Geometry check sheet. Reference: the model listing, model coordinates, mm. Face numbers are marked on the shaded views. A direction names the side the tool comes from. Give positions to 0.01 mm unless a question says otherwise; leave off trailing zeros. Loops run counter-clockwise (first coordinate to the right, second up) from the corner with the lowest first, then second, coordinate; pieces in that order, holes last. Notation, with made-up numbers: (-12.75, 21.5) -> (13.25, 21.5) arc R37 ccw to (13.25, 58.5) -> close; hole circle Ø1 at (71, 2.25). An arc over 180 degrees is marked (long way). One line per question, with ' | ' between items.
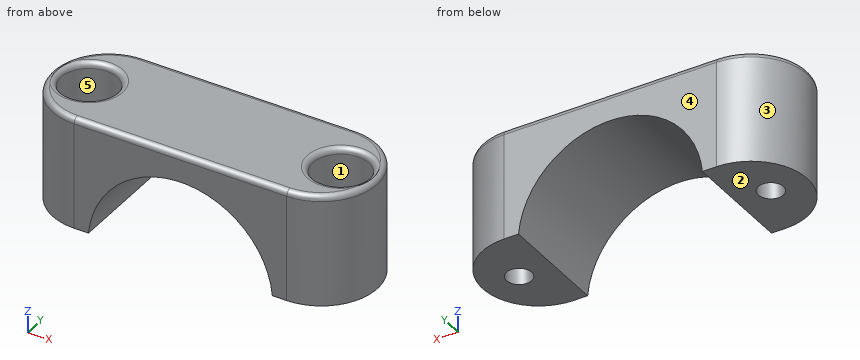
Autodesk Inventor part; units mm, degrees
ref_plane "YZ Plane" through (0, 0, 0) normal (1, 0, 0) x (0, 1, 0)
ref_plane "XZ Plane" through (0, 0, 0) normal (0, 1, 0) x (-1, 0, 0)
ref_plane "XY Plane" through (0, 0, 0) normal (0, 0, 1) x (1, 0, 0)
sketch "Sketch1" plane through (0, 0, 0) normal (0, 0, 1) x (1, 0, 0)
  line L0 (19, 10) -> (-19, 10)
  arc A0 (19, -10) -> (19, 10) centre (19, 0) ccw
  line L1 (-19, -10) -> (19, -10)
  arc A1 (-19, 10) -> (-19, -10) centre (-19, 0) ccw
  circle A2 centre (22.5, 0) radius 2.25
  circle A3 centre (-22.5, 0) radius 2.25
  point P0 (0, 0)
extrude "Extrusion1" add sketch "Sketch1" along normal blind 20 contours A0 L1 A1 L0 | A2 | A3
sketch "Sketch2" plane through (-19, -10, 0) normal (0, -1, 0) x (1, 0, 0)
  arc A0 (3, 0) -> (35, 0) centre (19, 0) ccw
  line L0 (3, 0) -> (0, 0)
  line L1 (0, -40) -> (0, 0)
  line L2 (0, -40) -> (38, -40)
  line L3 (38, -40) -> (38, 0)
  line L4 (38, 0) -> (35, 0)
  circle A1 centre (19, 0) radius 16
  line L5 (0, 0) -> (38, 0)
  line L6 (38, 0) -> (38, 20)
  line L7 (0, 20) -> (38, 20)
  line L8 (0, 0) -> (0, 20)
  point P0 (19, 0)
  point P1 (3, 0)
  point P2 (35, 0)
extrude "Extrusion2" cut sketch "Sketch2" against normal through all contours A1 L5
sketch "Sketch3" plane through (0, 0, 20) normal (0, 0, 1) x (1, 0, 0)
  arc A0 (-19, 10) -> (-19, -10) centre (-19, 0) ccw
  line L0 (-19, -10) -> (19, -10)
  arc A1 (19, -10) -> (19, 10) centre (19, 0) ccw
  line L1 (19, 10) -> (-19, 10)
  line L2 (-16, -10.4231) -> (-16, -76.7035)
  arc A2 (-19, 10) -> (-19, -10) centre (-19, 0) ccw
  line L3 (-29, 0) -> (-16, 0)
  circle A3 centre (-22.5, 0) radius 2.25
  line L4 (19, 10) -> (-19, 10)
  line L5 (0, 10) -> (0, -10)
  circle A4 centre (22.5, 0) radius 2.25
  line L6 (-22.5, 0) -> (-26, 0)
  line L7 (-26, 2.0207) -> (-22.5, 4.0415)
  line L8 (-22.5, 4.0415) -> (-19, 2.0207)
  line L9 (-19, 2.0207) -> (-19, -2.0207)
  line L10 (-19, -2.0207) -> (-22.5, -4.0415)
  line L11 (-22.5, -4.0415) -> (-26, -2.0207)
  line L12 (-26, -2.0207) -> (-26, 2.0207)
  line L13 (26, 2.0207) -> (22.5, 4.0415)
  line L14 (22.5, 4.0415) -> (19, 2.0207)
  line L15 (19, 2.0207) -> (19, -2.0207)
  line L16 (19, -2.0207) -> (22.5, -4.0415)
  line L17 (22.5, -4.0415) -> (26, -2.0207)
  line L18 (26, -2.0207) -> (26, 2.0207)
  point P0 (0, 0)
  dimension "d4" = 4.5
  dimension "d5" = 3.5
extrude "Extrusion3" [suppressed]
extrude "Extrusion4" cut sketch "Sketch3" against normal blind 5.5 contours L3 A3 | L3 A3 | A3 L3 L12 L7 L8 L9 | L3 L9 L10 L11 L12 A3 | A4 | L18 L17 L16 L15 L14 L13
extrude "Extrusion5" cut sketch "Sketch3" against normal through all contours L3 A3 | L3 A3 | A4
sketch "Sketch4" plane through (0, 0, 20) normal (0, 0, 1) x (1, 0, 0)
  line L0 (19, 2.0207) -> (22.5, 4.0415)
  line L1 (22.5, 4.0415) -> (26, 2.0207)
  line L2 (26, 2.0207) -> (26, -2.0207)
  line L3 (26, -2.0207) -> (22.5, -4.0415)
  line L4 (22.5, -4.0415) -> (19, -2.0207)
  line L5 (19, -2.0207) -> (19, 2.0207)
  line L6 (-19, -2.0207) -> (-22.5, -4.0415)
  line L7 (-22.5, -4.0415) -> (-26, -2.0207)
  line L8 (-26, -2.0207) -> (-26, 2.0207)
  line L9 (-26, 2.0207) -> (-22.5, 4.0415)
  line L10 (-22.5, 4.0415) -> (-19, 2.0207)
  line L11 (-19, 2.0207) -> (-19, -2.0207)
  arc A0 (-19, 10) -> (-19, -10) centre (-19, 0) ccw
  line L12 (-19, -10) -> (19, -10)
  arc A1 (19, -10) -> (19, 10) centre (19, 0) ccw
  line L13 (19, 10) -> (-19, 10)
  point P0 (0, 0)
extrude "Extrusion6" add sketch "Sketch4" along normal blind 1.5
sketch "Sketch5" plane through (0, 0, 0) normal (0, 0, -1) x (-1, 0, 0)
  circle A0 centre (-22.5, 0) radius 2.25
  line L0 (-16, -10) -> (-16, 10)
  line L1 (-19, 10) -> (-16, 10)
  arc A1 (-19, 10) -> (-19, -10) centre (-19, 0) ccw
  line L2 (-16, -10) -> (-19, -10)
  circle A2 centre (22.5, 0) radius 2.25
  line L3 (16, 10) -> (16, -10)
  line L4 (19, -10) -> (16, -10)
  arc A3 (19, -10) -> (19, 10) centre (19, 0) ccw
  line L5 (16, 10) -> (19, 10)
  point P0 (0, 0)
extrude "Extrusion7" cut sketch "Sketch5" against normal blind 0.5
sketch "Sketch6" plane through (0, -10, 0) normal (0, -1, 0) x (1, 0, 0)
  line L0 (-19, 0.5) -> (-19, 21.5)
  line L1 (-19, 0.5) -> (-16, 0.5)
  line L2 (-16, 0.5) -> (-16, 0)
  arc A0 (16, 0) -> (-16, 0) centre (0, 0) ccw
  line L3 (16, 0) -> (16, 0.5)
  line L4 (16, 0.5) -> (19, 0.5)
  line L5 (19, 0.5) -> (19, 21.5)
  arc A1 (16, 0) -> (-16, 0) centre (0, 0) ccw
  line L6 (0, 16) -> (0, 16.5)
  circle A2 centre (0, 0) radius 16.5
  line L7 (-19, 21.5) -> (19, 21.5)
  point P0 (0, 0)
  point P1 (16.4924, 0.5)
  point P2 (-16.4924, 0.5)
  dimension "d17" = 0.5
extrude "Extrusion8" cut sketch "Sketch6" against normal through all contours A2 L6 A0 L2 L1 | A2 L4 L3 A0 L6
sketch "Sketch7" plane through (0, 0, 21.5) normal (0, 0, 1) x (1, 0, 0)
  circle A0 centre (-22.5, 0) radius 2.25
  line L0 (-22.5, -4.0415) -> (-26, -2.0207)
  line L1 (-19, -2.0207) -> (-22.5, -4.0415)
  line L2 (-19, 2.0207) -> (-19, -2.0207)
  line L3 (-22.5, 4.0415) -> (-19, 2.0207)
  line L4 (-26, 2.0207) -> (-22.5, 4.0415)
  line L5 (-26, -2.0207) -> (-26, 2.0207)
  circle A1 centre (22.5, 0) radius 2.25
  line L6 (22.5, 4.0415) -> (26, 2.0207)
  line L7 (19, 2.0207) -> (22.5, 4.0415)
  line L8 (19, -2.0207) -> (19, 2.0207)
  line L9 (22.5, -4.0415) -> (19, -2.0207)
  line L10 (26, -2.0207) -> (22.5, -4.0415)
  line L11 (26, 2.0207) -> (26, -2.0207)
  point P0 (0, 0)
extrude "Extrusion9" cut sketch "Sketch7" against normal blind 15
sketch "Sketch8" plane through (0, 0, 21.5) normal (0, 0, 1) x (1, 0, 0)
  line L0 (-19, -10) -> (19, -10)
  arc A0 (19, -10) -> (19, 10) centre (19, 0) ccw
  line L1 (19, 10) -> (-19, 10)
  arc A1 (-19, 10) -> (-19, -10) centre (-19, 0) ccw
  line L2 (-19, -2.0207) -> (-22.5, -4.0415)
  line L3 (-22.5, -4.0415) -> (-26, -2.0207)
  line L4 (-26, -2.0207) -> (-26, 2.0207)
  line L5 (-26, 2.0207) -> (-22.5, 4.0415)
  line L6 (-22.5, 4.0415) -> (-19, 2.0207)
  line L7 (-19, 2.0207) -> (-19, -2.0207)
  line L8 (19, 2.0207) -> (22.5, 4.0415)
  line L9 (22.5, 4.0415) -> (26, 2.0207)
  line L10 (26, 2.0207) -> (26, -2.0207)
  line L11 (26, -2.0207) -> (22.5, -4.0415)
  line L12 (22.5, -4.0415) -> (19, -2.0207)
  line L13 (19, -2.0207) -> (19, 2.0207)
  circle A2 centre (-22.5, 0) radius 2.25
  circle A3 centre (22.5, 0) radius 2.25
  circle A4 centre (-22.5, 0) radius 5
  circle A5 centre (22.5, 0) radius 5
  point P0 (0, 0)
  dimension "d22" = 10
  dimension "d23" = 10
extrude "Extrusion10" cut sketch "Sketch8" against normal blind 11 contours L2 L3 L4 L5 L6 L7 | L8 L9 L10 L11 L12 L13 | A2 | A3 | A4 | A5
fillet "Fillet2" radius 1 6 edges at (0, -10, 21.5) (29, 0, 21.5) (0, 10, 21.5) (-29, 0, 21.5) (-27.5, 0, 21.5) (17.5, 0, 21.5)
sketch "Szkic9" plane through (0, 0, 6.5) normal (0, 0, 1) x (1, 0, 0)
  line L0 (-19, 2.0207) -> (-19, -2.0207)
  line L1 (-22.5, 4.0415) -> (-19, 2.0207)
  line L2 (-26, 2.0207) -> (-22.5, 4.0415)
  line L3 (-26, -2.0207) -> (-26, 2.0207)
  line L4 (-22.5, -4.0415) -> (-26, -2.0207)
  line L5 (-19, -2.0207) -> (-22.5, -4.0415)
  circle A0 centre (-22.5, 0) radius 2.25
  line L6 (19, -2.0207) -> (19, 2.0207)
  line L7 (22.5, -4.0415) -> (19, -2.0207)
  line L8 (26, -2.0207) -> (22.5, -4.0415)
  line L9 (26, 2.0207) -> (26, -2.0207)
  line L10 (22.5, 4.0415) -> (26, 2.0207)
  line L11 (19, 2.0207) -> (22.5, 4.0415)
  circle A1 centre (22.5, 0) radius 2.25
  point P0 (0, 0)
extrude "Wyciągnięcie proste11" cut sketch "Szkic9" against normal blind 1
sketch "Szkic10" plane through (0, 0, 0.5) normal (0, 0, -1) x (-1, 0, 0)
  line L0 (-16.4924, -10) -> (-16.4924, 10)
  line L1 (-19, 10) -> (-16.4924, 10)
  arc A0 (-19, 10) -> (-19, -10) centre (-19, 0) ccw
  line L2 (-16.4924, -10) -> (-19, -10)
  circle A1 centre (-22.5, 0) radius 2.25
  circle A2 centre (22.5, 0) radius 2.25
  line L3 (16.4924, 10) -> (16.4924, -10)
  line L4 (19, -10) -> (16.4924, -10)
  arc A3 (19, -10) -> (19, 10) centre (19, 0) ccw
  line L5 (16.4924, 10) -> (19, 10)
  point P0 (0, 0)
extrude "Wyciągnięcie proste12" cut sketch "Szkic10" against normal blind 1
sketch "Szkic11" plane through (-16.4924, -10, 0.5) normal (-1, 0, 0) x (0, 0, 1)
  line L0 (0, 20) -> (0, 0)
  line L1 (1, 0) -> (0, 0)
  line L2 (1, 0) -> (1, 20)
  line L3 (0, 20) -> (1, 20)
  point P0 (-0.5, 10)
extrude "Wyciągnięcie proste13" cut sketch "Szkic11" against normal through all
properties part number "Uchwyt_silnika_2_dół" material "Kauczuk"
Item 1: Set-up check for the marked faces 1 and 2: record each of +Z, -Z, +X, -X, +Y, -Y from which the full face is reachable in a straight line by a thin tool's end or side.
Result:
face 1: +Z | face 2: -Z, +X, -X, +Y, -Y
Item 2: Sectioned sample at C-C (x = 0). Record the cut outline in (y, z).
Result:
outline: (-10, 16.5) -> (10, 16.5) -> (10, 20.5) arc R1 ccw to (9, 21.5) -> (-9, 21.5) arc R1 ccw to (-10, 20.5) -> close
Item 3: Depth check by flat-ended pin: pin 1 Ø1.5 at (y, z) = (5.5, 4) entering from -X; pin 2 Ø5 at (x, y) = (-22, 2) entering from +Z; pin 3 Ø3.5 at (x, y) = (-22.5, 0) entering from +Z; pin 4 Ø3 at (x, y) = (-23, 1.5) entering from +Z. Enter the tip coordinate at first touch or a pass-through.
Result:
pin 1: x = -27.8 | pin 2: z = 10.5 | pin 3: through | pin 4: z = 5.5
Item 4: Sectioned sample at D-D (x = 12.5). Record the cut outline in (y, z).
Result:
outline: (-10, 10.77) -> (10, 10.77) -> (10, 20.5) arc R1 ccw to (9, 21.5) -> (-9, 21.5) arc R1 ccw to (-10, 20.5) -> close
Item 5: Sectioned sample at A-A (z = 11.25). Record the cut outline in (x, y).
Result:
outline: (-19, -10) -> (-12.07, -10) -> (-12.07, 10) -> (-19, 10) arc R10 ccw to start; (12.07, -10) -> (19, -10) arc R10 ccw to (19, 10) -> (12.07, 10) -> close; hole circle Ø10 at (-22.5, 0); hole circle Ø10 at (22.5, 0)
Item 6: Scan lines: probe 1 along X at (y, z) = (0.75, 5); probe 2 along X at (y, z) = (-4.25, 12.5); probe 3 along X at (y, z) = (-1.5, 20). Record each from-to range of solid material in increasing order.
Result:
probe 1: -28.97 to -24.62, -20.38 to -15.72, 15.72 to 20.38, 24.62 to 28.97 | probe 2: -28.05 to -25.13, -19.87 to -10.77, 10.77 to 19.87, 25.13 to 28.05 | probe 3: -28.89 to -27.27, -17.73 to 17.73, 27.27 to 28.89
Item 7: Sectioned sample at B-B (y = 0). Give the number of separate pieces and of enclosed holes in the cut face, plus the area to 3 significant figures.
Result:
separate pieces: 3 | enclosed holes: 0 | area: 455 mm2
Item 8: Release check for a two-part mould opening along Y. For the marked faces 3, 4 and 5 record: pulls with the +Y half, pulls with the -Y half, needs draft (parallel to the pull), parting line crosses it, or undercut.
Result:
face 3: parting line crosses it | face 4: pulls with the +Y half | face 5: undercut
